Part model, mm, in its own coordinate system. A direction names the side the tool comes from. Give positions to 0.01 mm unless a question says otherwise; leave off trailing zeros. Loops run counter-clockwise (first coordinate to the right, second up) from the corner with the lowest first, then second, coordinate; pieces in that order, holes last. Notation, with made-up numbers: (35, 9.5) -> (39, 9.5) arc R22 cw to (39, 19.5) -> close; hole circle Ø2 at (48.5, 47.5). An arc over 180 degrees is marked (long way). Write item = value, one per line.
from build123d import *

# Parameters (mm, degrees)
SKETCH1_W           = 38.1
SKETCH1_H           = 38.1
BOSS_EXTRUDE1_DEPTH = 25.4
SKETCH2_R           = 3.175
BOSS_EXTRUDE2_DEPTH = 12.7


with BuildPart() as part:
    # Sketch1 → Boss-Extrude1 (new, symmetric)
    with BuildSketch(Plane.XY):
        Rectangle(SKETCH1_W, SKETCH1_H)
    extrude(amount=BOSS_EXTRUDE1_DEPTH, both=True)

    # Sketch2 → Boss-Extrude2 (add)
    with BuildSketch(Plane.XY.offset(25.4)):
        with Locations(Location((0, 0, 0), (0, 0, 180))):
            Circle(SKETCH2_R)
    extrude(amount=BOSS_EXTRUDE2_DEPTH)


solid = part.part
1) Slice it at C-C, the plane z = 31.5. List the corners of the cut face in (x, y) (3 decimals), and give its area (3 significant figures).
Resolved:
outline = circle Ø6.35 at (0, 0)
area = 31.7 mm²
2) Slice it at D-D, the plane y = -7. List the corners of the cut face in (x, z).
Resolved:
outline = (-19.05, -25.4) -> (19.05, -25.4) -> (19.05, 25.4) -> (-19.05, 25.4) -> close
3) Which spindle directions (+Z, -Z, +X, -X, +Y, -Y) get a long thin tool onto all of the face, cutting with end or side? Do faces 1 (the face through (0, -19.05, 0)), 2 (the face through (-1.5, 2.8, 31.7)). Say none if no direction does.
Resolved:
face_1 = +Z, -Z, +X, -X, -Y
face_2 = +Z
4) Drill centre lines: line 1 along Z through (x, y) = (8, -13.5); line 2 along X through (y, z) = (-1, 31). Where is each one in solid material? Low to high. Write a range as [from, to].
Resolved:
line_1 = [-25.4, 25.4]
line_2 = [-3.01, 3.01]
5) Slice it at A-A, the plane x = 0. List the corners of the cut face in (y, z) (3 decimals).
Resolved:
outline = (-19.05, -25.4) -> (19.05, -25.4) -> (19.05, 25.4) -> (3.175, 25.4) -> (3.175, 38.1) -> (-3.175, 38.1) -> (-3.175, 25.4) -> (-19.05, 25.4) -> close
6) Drop flat-ended pins along their axis: P1, Ø12, axis at x = -8.5, y = -12, coming from the +Z side; P2, Ø3, axis at x = -8.5, z = 26.5, coming from the +Y side. Give the stop position or say it passes through.
Resolved:
P1 = 25.4
P2 = 19.05
